Input: part model. Units: mm. Frame: model coordinates. Face numbers are marked on the shaded views. Coordinates: 2 decimals unless noted, no trailing zeros. Order: outer loops, then holes, each group sorted by start corner. A loop starts at its lowest first (then second) coordinate and runs counter-clockwise, first axis right, second up. Notation, with made-up numbers: (53.5, 57) - (57.5, 57) arc R29 cw to (57.5, 90) - close; hole circle Ø4 at (-3.75, -7). An arc over 180 degrees is marked (long way). Use a Markdown table: item, result. Add a question column.
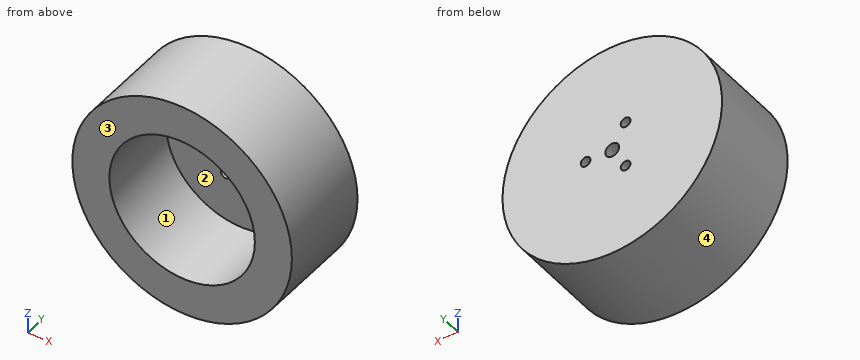
from build123d import *

# Parameters (mm, degrees)
SKETCH_1_R          = 35
EXTRUDE_1_DEPTH     = 30
SKETCH_2_R          = 23.2
CUT_EXTRUDE_1_DEPTH = 26
CUT_EXTRUDE_2_REACH = 32
SKETCH_3_R          = 2.2
SKETCH_3_R_2        = 1.55


with BuildPart() as part:
    # 草图1 → 凸台-拉伸1 (new body)
    with BuildSketch(Plane(origin=(0, 0, 0), x_dir=(1, 0, 0), z_dir=(0, 1, 0))):
        Circle(SKETCH_1_R)
    extrude(amount=EXTRUDE_1_DEPTH)

    # 草图2 → 切除-拉伸1 (cut)
    with BuildSketch(Plane.XZ):
        Circle(SKETCH_2_R)
    extrude(amount=-CUT_EXTRUDE_1_DEPTH, mode=Mode.SUBTRACT)

    # 草图3 → 切除-拉伸2 (cut, up to next)
    with BuildSketch(Plane(origin=(0, 30, 0), x_dir=(1, 0, 0), z_dir=(0, 1, 0)), mode=Mode.PRIVATE) as cut_extrude_2_sk1:
        Circle(SKETCH_3_R)
    cut_extrude_2_tool1 = extrude(cut_extrude_2_sk1.sketch, amount=-CUT_EXTRUDE_2_REACH, mode=Mode.PRIVATE) & part.part
    add(cut_extrude_2_tool1.solids().sort_by_distance((0, 30, 0))[0], mode=Mode.SUBTRACT)
    # 草图3 → 切除-拉伸2 (cut, up to next)
    with BuildSketch(Plane(origin=(0, 30, 0), x_dir=(1, 0, 0), z_dir=(0, 1, 0)), mode=Mode.PRIVATE) as cut_extrude_2_sk2:
        with Locations((8.5, 0)):
            Circle(SKETCH_3_R_2)
    cut_extrude_2_tool2 = extrude(cut_extrude_2_sk2.sketch, amount=-CUT_EXTRUDE_2_REACH, mode=Mode.PRIVATE) & part.part
    add(cut_extrude_2_tool2.solids().sort_by_distance((8.5, 30, 0))[0], mode=Mode.SUBTRACT)
    # 草图3 → 切除-拉伸2 (cut, up to next)
    with BuildSketch(Plane(origin=(0, 30, 0), x_dir=(1, 0, 0), z_dir=(0, 1, 0)), mode=Mode.PRIVATE) as cut_extrude_2_sk3:
        with Locations((-4.25, -7.361215932)):
            Circle(SKETCH_3_R_2)
    cut_extrude_2_tool3 = extrude(cut_extrude_2_sk3.sketch, amount=-CUT_EXTRUDE_2_REACH, mode=Mode.PRIVATE) & part.part
    add(cut_extrude_2_tool3.solids().sort_by_distance((-4.25, 30, 7.361216))[0], mode=Mode.SUBTRACT)
    # 草图3 → 切除-拉伸2 (cut, up to next)
    with BuildSketch(Plane(origin=(0, 30, 0), x_dir=(1, 0, 0), z_dir=(0, 1, 0)), mode=Mode.PRIVATE) as cut_extrude_2_sk4:
        with Locations((-4.25, 7.361215932)):
            Circle(SKETCH_3_R_2)
    cut_extrude_2_tool4 = extrude(cut_extrude_2_sk4.sketch, amount=-CUT_EXTRUDE_2_REACH, mode=Mode.PRIVATE) & part.part
    add(cut_extrude_2_tool4.solids().sort_by_distance((-4.25, 30, -7.361216))[0], mode=Mode.SUBTRACT)


solid = part.part
1) Contact query for flat-ended pins moving along their axis: P1, Ø14, axis at x = -9.5, z = -1, coming from the -Y side; P2, Ø1.5, axis at y = 19, z = -20.5, coming from the +X side; P3, Ø1.5, axis at y = 11.5, z = -16.5, coming from the -X side. Output: stop coordinate, or through.
2) Cut plane B-B (x = 0). Return the cut outline in (y, z).
3) Material intervals for L1, parallel to X at y = 28.05, z = 0; L2, parallel to Z at x = 0, y = 13.5; L3, parallel to Y at x = -9, z = -7.5, sorted ascending.
4) Cut plane C-C (y = 11.75). Return the cut outline in (x, z), and give its area (3 significant figures).
5) Cut plane D-D (x = -21.5). Return the cut outline in (y, z), and give its area (3 significant figures).
6) Cut plane A-A (z = 0). Return the cut outline in (x, y), and give its area (3 significant figures).
7) Pull-direction query (Z, two-part tool) for the marked faces 1, 2, 3 and 4; classes: pulls with the +Z half, pulls with the -Z half, needs draft (parallel to the pull), parting line crosses it, or undercut.
Computed:
| question | item | result |
|---|---|---|
| 1 | P1 | stops at y = 26 |
| 1 | P2 | stops at x = 28.9 |
| 1 | P3 | stops at x = -31.26 |
| 2 | outline | (0, -35) - (30, -35) - (30, -2.2) - (26, -2.2) - (26, -23.2) - (0, -23.2) - close; (0, 23.2) - (26, 23.2) - (26, 2.2) - (30, 2.2) - (30, 35) - (0, 35) - close |
| 3 | L1 | x = -35 to -2.2, 2.2 to 6.95, 10.05 to 35 |
| 3 | L2 | z = -35 to -23.2, 23.2 to 35 |
| 3 | L3 | y = 26 to 30 |
| 4 | outline | circle Ø70 at (0, 0); hole circle Ø46.4 at (0, 0) |
| 4 | area | 2,160 mm2 |
| 5 | outline | (0, -27.62) - (30, -27.62) - (30, 27.62) - (0, 27.62) - (0, 8.72) - (26, 8.72) - (26, -8.72) - (0, -8.72) - close |
| 5 | area | 1,200 mm2 |
| 6 | outline | (-35, 0) - (-23.2, 0) - (-23.2, 26) - (-2.2, 26) - (-2.2, 30) - (-35, 30) - close; (2.2, 26) - (6.95, 26) - (6.95, 30) - (2.2, 30) - close; (10.05, 26) - (23.2, 26) - (23.2, 0) - (35, 0) - (35, 30) - (10.05, 30) - close |
| 6 | area | 864 mm2 |
| 7 | face 1 | undercut |
| 7 | face 2 | undercut |
| 7 | face 3 | needs draft |
| 7 | face 4 | parting line crosses it |
